Job drawing, mm, ordinate dimensions from the low corner. One solid piece. A direction names the side the tool comes from. Coordinates: 2 decimals unless noted, no trailing zeros. Order: outer loops, then holes, each group sorted by start corner. A loop starts at its lowest first (then second) coordinate and runs counter-clockwise, first axis right, second up. Notation, with made-up numbers: (37.5, 49.25) - (90.5, 49.25) arc R16 ccw to (90.5, 79.25) - close; hole circle Ø2 at (18, 68). An arc over 180 degrees is marked (long way). Use a Markdown table: item, result. Add a question column.
1) Saw through at D-D on y = 11.25. List the corners of the cut face in (x, z), then the cut area to 3 significant figures.
2) Drop a flat-ended pin along its axis: P1, Ø1, axis at x = 16, y = 12, coming from the +Z side. Give the stop position or say it passes through.
3) Saw through at A-A on z = 22. List the corners of the cut face in (x, y).
4) Saw through at C-C on y = 23.5. List the corners of the cut face in (x, z), then the cut area to 3 significant figures.
5) Saw through at B-B on x = 12. List the corners of the cut face in (y, z), then the cut area to 3 significant figures.
6) Tool access for the marked faces 1, 2 and 3: list every direction of +Z, -Z, +X, -X, +Y, -Y with a clear straight run to the whole face (end or side of a thin tool).
7) Wall check: L1, parallel to Z at x = 33.5, y = 1.75; L2, parallel to Y at x = 17, z = 25.5; L3, parallel to Y at x = 39.5, z = 22. Give the ranges that are in metal, low to high. Write a range as [from, to].
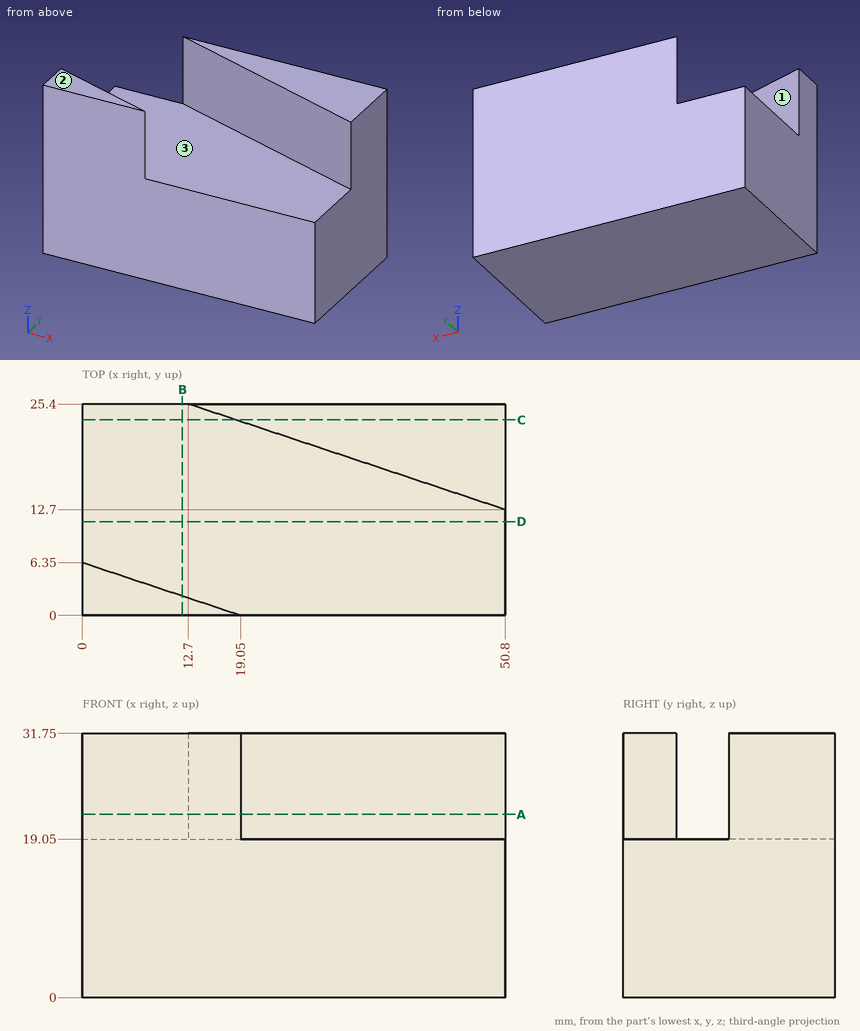
Results are:
| question | item | result |
|---|---|---|
| 1 | outline | (0, 0) - (50.8, 0) - (50.8, 19.05) - (0, 19.05) - close |
| 1 | area | 968 mm2 |
| 2 | P1 | z = 19.05 |
| 3 | outline | (0, 0) - (19.05, 0) - (0, 6.35) - close; (12.7, 25.4) - (50.8, 12.7) - (50.8, 25.4) - close |
| 4 | outline | (0, 0) - (50.8, 0) - (50.8, 31.75) - (18.4, 31.75) - (18.4, 19.05) - (0, 19.05) - close |
| 4 | area | 1,380 mm2 |
| 5 | outline | (0, 0) - (25.4, 0) - (25.4, 19.05) - (2.35, 19.05) - (2.35, 31.75) - (0, 31.75) - close |
| 5 | area | 514 mm2 |
| 6 | face 1 | +Z, +X |
| 6 | face 2 | +Z, +X, -X, +Y, -Y |
| 6 | face 3 | +Z |
| 7 | L1 | [0, 19.05] |
| 7 | L2 | [0, 0.68], [23.97, 25.4] |
| 7 | L3 | [16.47, 25.4] |
